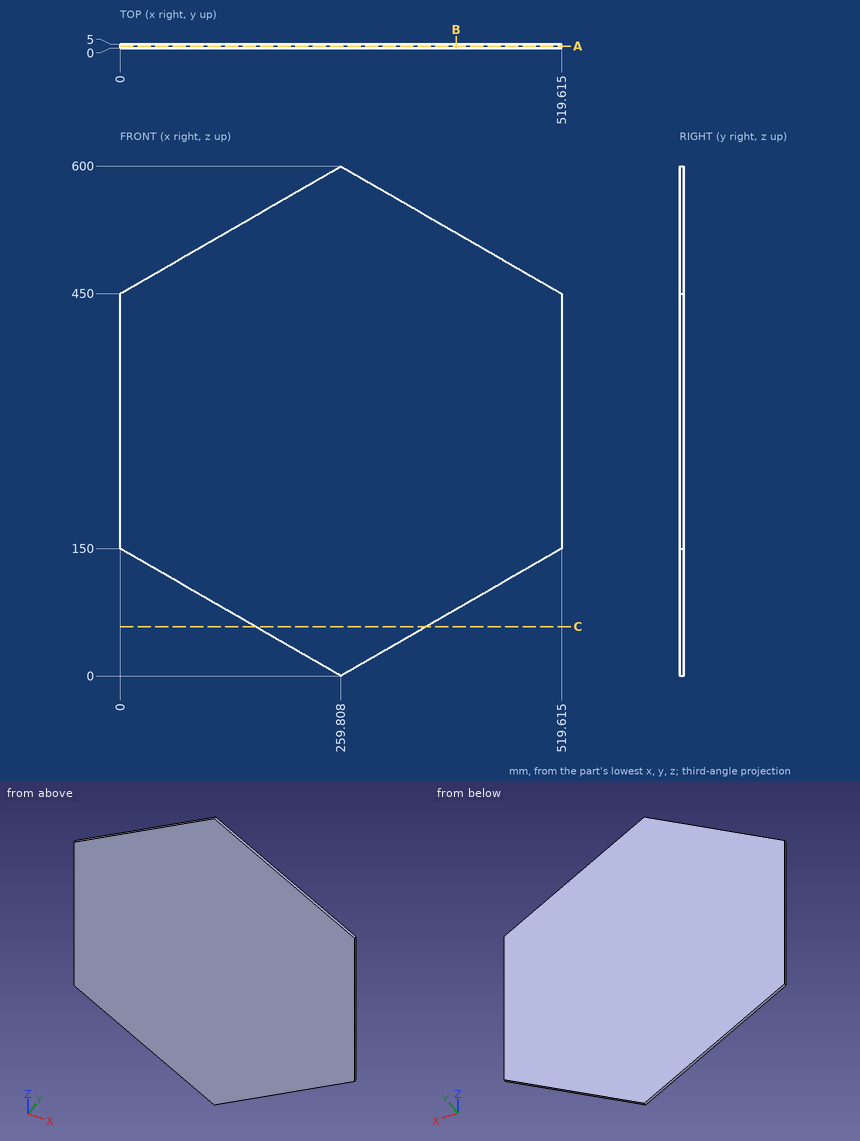
Could you check a few things on this drawing? It's one solid part, dimensions in mm from its lowest x, y, z. Coordinates: 2 decimals unless noted, no trailing zeros. Write each loop counter-clockwise with the first axis right and the second up, starting at its lowest first coordinate (ties: lowest second). Pieces come first, ordered by that corner, then holes. Notation, with made-up numbers: (-31, -18.5) - (22, -18.5) arc R11 cw to (22, -3.5) - close; hole circle Ø10 at (44.5, 10). An arc over 180 degrees is marked (long way). Return JSON: item names as keys, results as strings. Group by question number.
Item 1: I'm going to push flat-ended pins straight in: pin 1 Ø1.5 at (y, z) = (3, 137) entering from -X; pin 2 Ø2 at (x, y) = (454, 2) entering from +Z. Where does each tip first touch, or does it pass through?
Item 2: If we section it at B-B (x = 395.5): Write out the boundary of the cut face in (y, z), then the cut area to 3 significant figures.
Item 3: Please list where these lines run through material, in increasing order: probe 1 along Z at (x, y) = (282.5, 1.9); probe 2 along Z at (x, y) = (338, 0.4) (1 decimal); probe 3 along X at (y, z) = (3.3, 105) (1 decimal).
Item 4: If we section it at C-C (z = 58): Write out the boundary of the cut face in (x, y).
Item 5: If we section it at A-A (y = 2.4): Write out the boundary of the cut face in (x, z) (1 decimal).
Return value:
{
 "1": {"pin 1": "stops at x = 21.22", "pin 2": "stops at z = 488.46"},
 "2": {"outline": "(0, 78.34) - (5, 78.34) - (5, 521.66) - (0, 521.66) - close", "area": "2,220 mm^2"},
 "3": {"probe 1": "z = 13.1 to 586.9", "probe 2": "z = 45.1 to 554.9", "probe 3": "x = 77.9 to 441.7"},
 "4": {"outline": "(159.35, 0) - (360.27, 0) - (360.27, 5) - (159.35, 5) - close"},
 "5": {"outline": "(0, 150) - (259.8, 0) - (519.6, 150) - (519.6, 450) - (259.8, 600) - (0, 450) - close"}
}
